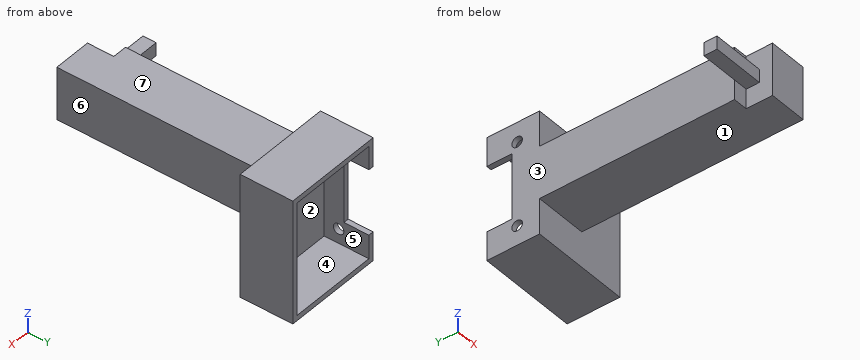
from build123d import *

# Parameters (mm, degrees)
SKETCH3_W            = 38
SKETCH3_H            = 47
SKETCH3_W_2          = 34
SKETCH3_H_2          = 43
BOSS_EXTRUDE4_DEPTH  = 10.5
SKETCH1_W            = 34
SKETCH1_H            = 43
BOSS_EXTRUDE5_DEPTH  = 3
BOSS_EXTRUDE6_DEPTH  = 9.5
CUT_EXTRUDE1_REACH   = 4
SKETCH6_R            = 2
SKETCH8_W            = 20
SKETCH8_H            = 20
BOSS_EXTRUDE7_DEPTH  = 84
CUT_EXTRUDE2_DEPTH   = 5.5
SKETCH12_W           = 5
SKETCH12_H           = 5
BOSS_EXTRUDE11_DEPTH = 14.5


with BuildPart() as part:
    # Sketch3 → Boss-Extrude4 (new body)
    with BuildSketch(Plane(origin=(0, 0, 0), x_dir=(1, 0, 0), z_dir=(0, 1, 0))):
        with Locations((31, 71.5)):
            Rectangle(SKETCH3_W, SKETCH3_H)
        with Locations((31, 71.5)):
            Rectangle(SKETCH3_W_2, SKETCH3_H_2, mode=Mode.SUBTRACT)
    extrude(amount=BOSS_EXTRUDE4_DEPTH)

    # Sketch1 → Boss-Extrude5 (add)
    with BuildSketch(Plane(origin=(0, 0, 0), x_dir=(1, 0, 0), z_dir=(0, 1, 0))):
        with Locations((31, 71.5)):
            Rectangle(SKETCH1_W, SKETCH1_H)
    extrude(amount=BOSS_EXTRUDE5_DEPTH)

    # Sketch7 → Boss-Extrude6 (add)
    with BuildSketch(Plane(origin=(0, 10.5, 0), x_dir=(1, 0, 0), z_dir=(0, 1, 0))):
        Polygon((14, 50), (14, 59), (12, 59), (12, 48), (50, 48), (50, 95), (12, 95), (12, 84), (14, 84), (14, 93), (48, 93), (48, 50), align=None)
    extrude(amount=BOSS_EXTRUDE6_DEPTH)

    # Sketch6 → Cut-Extrude1 (cut, up to next)
    with BuildSketch(Plane(origin=(14, 0, 0), x_dir=(0, 0, -1), z_dir=(1, 0, 0)), mode=Mode.PRIVATE) as cut_extrude1_sk1:
        with Locations((55.5, 8.5)):
            Circle(SKETCH6_R)
    cut_extrude1_tool1 = extrude(cut_extrude1_sk1.sketch, amount=-CUT_EXTRUDE1_REACH, mode=Mode.PRIVATE) & part.part
    add(cut_extrude1_tool1.solids().sort_by_distance((14, 8.5, -55.5))[0], mode=Mode.SUBTRACT)
    # Sketch6 → Cut-Extrude1 (cut, up to next)
    with BuildSketch(Plane(origin=(14, 0, 0), x_dir=(0, 0, -1), z_dir=(1, 0, 0)), mode=Mode.PRIVATE) as cut_extrude1_sk2:
        with Locations((87.5, 8.5)):
            Circle(SKETCH6_R)
    cut_extrude1_tool2 = extrude(cut_extrude1_sk2.sketch, amount=-CUT_EXTRUDE1_REACH, mode=Mode.PRIVATE) & part.part
    add(cut_extrude1_tool2.solids().sort_by_distance((14, 8.5, -87.5))[0], mode=Mode.SUBTRACT)

    # Sketch8 → Boss-Extrude7 (add)
    with BuildSketch(Plane.XZ):
        with Locations((22, -71.5)):
            Rectangle(SKETCH8_W, SKETCH8_H)
    extrude(amount=BOSS_EXTRUDE7_DEPTH)

    # Sketch11 → Cut-Extrude2 (cut)
    with BuildSketch(Plane.ZY.offset(-12)):
        Polygon((-74, -74), (-81.5, -74), (-81.5, -84), (-61.5, -84), (-61.5, -74), (-69, -74), (-69, -79), (-74, -79), align=None)
    extrude(amount=-CUT_EXTRUDE2_DEPTH, mode=Mode.SUBTRACT)

    # Sketch12 → Boss-Extrude11 (add)
    with BuildSketch(Plane.ZY.offset(-12)):
        with Locations((-71.5, -76.5)):
            Rectangle(SKETCH12_W, SKETCH12_H)
    extrude(amount=BOSS_EXTRUDE11_DEPTH)


solid = part.part
Here's how the part is built. I have some questions about the finished solid (model axes, mm). Face numbers are marked on the shaded views. A direction names the side the tool comes from. Give positions to 0.01 mm unless a question says otherwise; leave off trailing zeros. Order: outer loops, then holes, each group sorted by start corner. A loop starts at its lowest first (then second) coordinate and runs counter-clockwise, first axis right, second up. Notation, with made-up numbers: (-10, -32.5) -> (3, -32.5) arc R33 ccw to (3, -1.5) -> close; hole circle Ø3 at (-15, 44.25). An arc over 180 degrees is marked (long way). One line per item, written item: value. Start each with the question number.
1. Imagine slicing it at B-B, the plane z = -55.5. List the corners of the cut face in (x, y) for me.
2. Will these pins go through, and if not, where does the flat tip stop? pin 1 Ø4 at (x, y) = (12, -76.5) entering from +Z; pin 2 Ø1.5 at (x, y) = (2.5, -76.5) entering from -Z; pin 3 Ø16 at (x, y) = (25.5, -48.5) entering from +Z; pin 4 Ø12 at (x, y) = (5, -30.5) entering from -Z.
3. Imagine slicing it at C-C, the plane x = 26.5. List the corners of the cut face in (y, z) for me, plus the area to 3 significant figures.
4. I need wall thicknesses on probe 1 along Y at (x, z) = (12.8, -87.5); probe 2 along X at (y, z) = (4.5, -56); probe 3 along Z at (x, y) = (13, 8). Which ranges of each line are inside material? Lowest first, please. Write a range as from..to.
5. Imagine slicing it at D-D, the plane y = -60.5. List the corners of the cut face in (x, z) for me.
6. Imagine slicing it at A-A, the plane y = 8.5. List the corners of the cut face in (x, z) for me, plus the area to 3 significant figures.
7. For the marked faces 1, 2 and 3, which set-ups out of +Z, -Z, +X, -X, +Y, -Y let a thin tool reach every point of the face, with its end or its side?
8. We'd pull the mould along X, two halves only. Please class the marked faces 4, 5, 6 and 7: released by +X, released by -X, zero draft, split by the parting line, or undercut.
Values follow:
1. outline: (12, 0) -> (50, 0) -> (50, 20) -> (48, 20) -> (48, 3) -> (14, 3) -> (14, 6.5) -> (12, 6.5) -> close; (12, 10.5) -> (14, 10.5) -> (14, 20) -> (12, 20) -> close
2. pin 1: stops at z = -69
2. pin 2: stops at z = -74
2. pin 3: stops at z = -61.5
2. pin 4: passes through
3. outline: (-84, -81.5) -> (0, -81.5) -> (0, -95) -> (20, -95) -> (20, -93) -> (3, -93) -> (3, -50) -> (20, -50) -> (20, -48) -> (0, -48) -> (0, -61.5) -> (-84, -61.5) -> close
3. area: 1,890 mm2
4. probe 1: y = 0..6.5, 10.5..20
4. probe 2: x = 12..14, 48..50
4. probe 3: z = -95..-89.44, -85.56..-57.44, -53.56..-48
5. outline: (12, -81.5) -> (32, -81.5) -> (32, -61.5) -> (12, -61.5) -> close
6. outline: (12, -95) -> (50, -95) -> (50, -48) -> (12, -48) -> (12, -53.5) -> (14, -53.5) -> (14, -50) -> (48, -50) -> (48, -93) -> (14, -93) -> (14, -89.5) -> (12, -89.5) -> close; (12, -85.5) -> (14, -85.5) -> (14, -57.5) -> (12, -57.5) -> close
6. area: 308 mm2
7. face 1: -Z, +X, -X, -Y
7. face 2: +Y
7. face 3: +Z, -Z, -X, +Y
8. face 4: undercut
8. face 5: undercut
8. face 6: released by +X
8. face 7: zero draft
